from build123d import *

# Parameters (mm, degrees)
SKETCH1_W           = 42
SKETCH1_H           = 20
BOSS_EXTRUDE1_DEPTH = 1
SKETCH2_R           = 4.027938591
SKETCH2_R_2         = 4.182706726
BOSS_EXTRUDE2_DEPTH = 15
SKETCH3_W           = 11.745093392
SKETCH3_H           = 3.800746796
SKETCH3_W_2         = 11.743469105
SKETCH3_H_2         = 12.98355877
BOSS_EXTRUDE3_DEPTH = 7


with BuildPart() as part:
    # Sketch1 → Boss-Extrude1 (new body)
    with BuildSketch(Plane.XY):
        with Locations((-4.931174089, -4.708502024)):
            Rectangle(SKETCH1_W, SKETCH1_H)
    extrude(amount=BOSS_EXTRUDE1_DEPTH)

    # Sketch2 → Boss-Extrude2 (add)
    with BuildSketch(Plane.XY):
        with Locations((-20.961145163, 0)):
            Circle(SKETCH2_R)
        with Locations((10.49307608, -8.234663003)):
            Circle(SKETCH2_R_2)
    extrude(amount=-BOSS_EXTRUDE2_DEPTH)

    # Sketch3 → Boss-Extrude3 (add)
    with BuildSketch(Plane.XY):
        with Locations((-7.305637446, 2.527727406)):
            Rectangle(SKETCH3_W, SKETCH3_H)
        with Locations((-7.30644959, -6.491779385)):
            Rectangle(SKETCH3_W_2, SKETCH3_H_2)
    extrude(amount=-BOSS_EXTRUDE3_DEPTH)


solid = part.part
The model under review builds one solid part; all positions refer to its coordinate system, in mm. A direction names the side the tool comes from. Round coordinates to 2 decimals unless told otherwise and drop trailing zeros. Loops run counter-clockwise (first coordinate to the right, second up) from the corner with the lowest first, then second, coordinate; pieces in that order, holes last. Notation, with made-up numbers: (-6, 82.25) -> (17, 82.25) arc R14 cw to (17, 107.25) -> close; hole circle Ø4 at (-24.75, 59). An arc over 180 degrees is marked (long way). Return JSON: item names as keys, results as strings.
(1) The part is to be moulded in two halves that separate along X. For faces 1 (the flat face through (16.069, -4.8, 0.5)), 2 (the cylindrical face through (-17.12, 1.21, -7.4)), 3 (the cylindrical face through (6.314, -8.051, -7.395)), 4 (the flat face through (-21, 0, -15)), say which applies: released by +X, released by -X, zero draft, split by the parting line, or undercut.
Solved:
{"face 1": "released by +X", "face 2": "undercut", "face 3": "undercut", "face 4": "zero draft"}
(2) For pin 1 (2 mm diameter, centred on y = -10, z = -10, fed in from +X); pin 2 (10 mm diameter, centred on x = -4.5, y = -7.5, fed in from -Z); pin 3 (3 mm diameter, centred on y = -12.5, z = -9, fed in from -X), all flat-tipped, find the tip position at first contact; note any pin that passes through.
Solved:
{"pin 1": "x = 14.61", "pin 2": "z = -7", "pin 3": "x = 7.35"}
(3) For faces 5 (the flat face through (-7, -12.984, -3)), 6 (the flat face through (-7, 4.428, -3)), 7 (the flat face through (-7, -6, -7)), list the 3-axis set-ups (+Z, -Z, +X, -X, +Y, -Y) from which the entire face can be reached by the end or side of a thin tool; tool diameter is ignored.
Solved:
{"face 5": "-Z, +X, -X, -Y", "face 6": "-Z, +X, -X, +Y", "face 7": "-Z, +Y, -Y"}
(4) For line 1 (Y direction, x = -13, z = -5.25); line 2 (Z direction, x = -19.5, y = -8.75); line 3 (Z direction, x = -2, y = -10), list the stretches that pass through material, from the lowest coordinate up.
Solved:
{"line 1": "-12.98 to 0, 0.63 to 4.43", "line 2": "0 to 1", "line 3": "-7 to 1"}
(5) Add section D-D on z = -9.75. Write out the cut boundary in (x, y).
Solved:
{"outline": "circle Ø8.06 at (-20.96, 0); circle Ø8.37 at (10.49, -8.23)"}
(6) Add section A-A on z = -4.5. Write out the cut boundary in (x, y), plus the area to 3 significant figures.
Solved:
{"outline": "circle Ø8.06 at (-20.96, 0); (-13.18, -12.98) -> (-1.43, -12.98) -> (-1.43, 0) -> (-13.18, 0) -> close; (-13.18, 0.63) -> (-1.43, 0.63) -> (-1.43, 4.43) -> (-13.18, 4.43) -> close; circle Ø8.37 at (10.49, -8.23)", "area": "303 mm2"}
(7) Add section B-B on y = -4.75. Write out the cut boundary in (x, z).
Solved:
{"outline": "(-25.93, 0) -> (-13.18, 0) -> (-13.18, -7) -> (-1.43, -7) -> (-1.43, 0) -> (8.18, 0) -> (8.18, -15) -> (12.81, -15) -> (12.81, 0) -> (16.07, 0) -> (16.07, 1) -> (-25.93, 1) -> close"}
(8) Add section C-C on x = -21. Write out the cut boundary in (y, z), plus the area to 3 significant figures.
Solved:
{"outline": "(-14.71, 0) -> (-4.03, 0) -> (-4.03, -15) -> (4.03, -15) -> (4.03, 0) -> (5.29, 0) -> (5.29, 1) -> (-14.71, 1) -> close", "area": "141 mm2"}
